Read the model definition and answer for the solid it produces. Units are mm, in the model's axes. A direction names the side the tool comes from. Round coordinates to 2 decimals unless told otherwise and drop trailing zeros. Order: outer loops, then holes, each group sorted by start corner. A loop starts at its lowest first (then second) coordinate and runs counter-clockwise, first axis right, second up. Notation, with made-up numbers: (-18.75, 35.25) -> (36.25, 35.25) arc R12 ccw to (36.25, 58.25) -> close; hole circle Ø8 at (53.5, -26.75). An arc over 180 degrees is marked (long way). Answer as a JSON object with one key per item and string values. Group by question number.
Item 1: Section D-D, the plane x = 59 is taken. Write down the section's boundary in (y, z).
Item 2: Section A-A, the plane z = 55 is taken. Write down the section's boundary in (x, y).
Item 3: Given P1, Ø2.5, axis at y = -5.1, z = 46.17, coming from the -X side; P2, Ø3, axis at x = -16.5, y = 42.5, coming from the -Z side; P3, Ø3, axis at x = -42.5, y = -17.6, coming from the +Z side, each flat-ended and moving along its own axis, determine where each tip first touches the part or whether it passes through.
Item 4: For faces 1 (the flat face through (16, 43, 2)), 2 (the cylindrical face through (-49, -48, 3)), 3 (the flat face through (85, -1, 76)), determine the directions among +Z, -Z, +X, -X, +Y, -Y from which every point of the face is accessible in a straight line to the end or side of a thin tool.
Item 5: Section C-C, the plane x = -25.5 is taken. Write down the section's boundary in (y, z).
Item 6: Section B-B, the plane x = 0 is taken. Write down the section's boundary in (y, z), plus the area to 3 significant figures.
Item 7: The mould has two halves that part along Z. Classify faces 4 (the flat face through (87, 1, 105)), 5 (the flat face through (-42, 16, 2)), 6 (the cylindrical face through (18.25, 39.57, 0.99)), 7 (the cylindrical face through (87.5, -4.3, 62)): pulls with the +Z half, pulls with the -Z half, needs draft (parallel to the pull), parting line crosses it, or undercut.
Item 8: Consider probe 1 along Y at (x, z) = (87, 55); probe 2 along Z at (x, y) = (47, -35); probe 3 along X at (y, z) = (-45.5, 28.5). Determine where each line is inside the solid, lowest interval first. Write a range as from..to.
Autodesk Inventor part; units mm, degrees
ref_plane "YZ Plane" through (0, 0, 0) normal (1, 0, 0) x (0, 1, 0)
ref_plane "XZ Plane" through (0, 0, 0) normal (0, 1, 0) x (-1, 0, 0)
ref_plane "XY Plane" through (0, 0, 0) normal (0, 0, 1) x (1, 0, 0)
sketch "スケッチ1" plane through (0, 0, 0) normal (0, 0, 1) x (1, 0, 0)
  circle A0 centre (0, 0) radius 48.5
  circle A1 centre (0, 0) radius 46.0893
  line L0 (-50, 50) -> (50, 50)
  line L1 (50, 50) -> (50, -50)
  line L2 (50, -50) -> (-50, -50)
  line L3 (-50, -50) -> (-50, 50)
  dimension "d0" = 97
  dimension "d3" = 50
  dimension "d4" = 50
  dimension "d5" = 50
  dimension "d6" = 50
extrude "押し出し1" add sketch "スケッチ1" along normal blind 5 contours A0 | A1 | L0 L1 L2 L3
sketch "スケッチ2" plane through (0, 0, 5) normal (0, 0, 1) x (1, 0, 0)
  circle A0 centre (0, 0) radius 46
  line L0 (0, 0) -> (0, 64.6511)
  line L1 (0, 0) -> (-25.9524, 62.6547)
  line L2 (-50, 50) -> (-50, -50)
  point P0 (-17.6034, 42.4985)
  point P1 (-42.4985, 17.6034)
  point P2 (-42.4985, -17.6034)
  point P3 (-17.6034, -42.4985)
  point P4 (17.6034, -42.4985)
  point P5 (42.4985, -17.6034)
  point P6 (42.4985, 17.6034)
  point P7 (17.6034, 42.4985)
  dimension "d7" = 92
  dimension "d8" = 22.5
  dimension "d11" = 360
  dimension "d76" = 50
hole "穴1" at (-17.6034, 42.4985, 5) at (-42.4985, 17.6034, 5) at (-42.4985, -17.6034, 5) at (-17.6034, -42.4985, 5) at (17.6034, -42.4985, 5) at (42.4985, -17.6034, 5) at (42.4985, 17.6034, 5) at (17.6034, 42.4985, 5) direction (0, 0, -1) diameter 2.459 end through all
sketch "スケッチ3" plane through (0, 0, 5) normal (0, 0, 1) x (1, 0, 0)
  circle A0 centre (0, 0) radius 30
  dimension "d20" = 60
extrude "押し出し2" cut sketch "スケッチ3" against normal blind 5
sketch "スケッチ4" plane through (50, -50, 0) normal (1, 0, 0) x (0, 0, -1)
  line L0 (-5, 100) -> (-5, 0)
  line L1 (-5, 100) -> (0, 100)
  line L2 (0, 100) -> (0, 0)
  line L3 (0, 0) -> (-5, 0)
  line L4 (-5, 0) -> (-5, 100)
  point P0 (0, 50)
extrude "押し出し3" add sketch "スケッチ4" along normal blind 40
sketch "スケッチ5" plane through (0, 0, 5) normal (0, 0, 1) x (1, 0, 0)
  line L0 (-50, 50) -> (90, 50)
  line L1 (85, 50) -> (90, 50)
  line L2 (90, 50) -> (90, -50)
  line L3 (90, -50) -> (85, -50)
  line L4 (85, -50) -> (85, 50)
  line L5 (-50, -50) -> (90, -50)
  line L6 (90, 50) -> (90, -50)
  point P0 (0, 0)
  point P1 (90, 50)
  point P2 (90, 0)
  dimension "d25" = 0
  dimension "d26" = 5
  dimension "d27" = 100
  dimension "d70" = 0
extrude "押し出し4" add sketch "スケッチ5" along normal blind 100
sketch "スケッチ6" plane through (90, -50, 0) normal (1, 0, 0) x (0, 0, -1)
  circle A0 centre (-55, 50) radius 46
  line L0 (0, 0) -> (-105, 0)
  line L1 (0, 0) -> (0, 100)
  line L2 (-55, 50) -> (41.9537, 50)
  line L3 (-55, 50) -> (-55, 131.7305)
  line L4 (-55, 50) -> (-80.0101, 110.3797)
  circle A1 centre (-55, 50) radius 12.5
  line L5 (-55, 50) -> (-63.1841, 64.1753)
  point P0 (0, 50)
  point P1 (-72.6034, 92.4985)
  point P2 (-97.4985, 67.6034)
  point P3 (-97.4985, 32.3966)
  point P4 (-72.6034, 7.5015)
  point P5 (-37.3966, 7.5015)
  point P6 (-12.5015, 32.3966)
  point P7 (-12.5015, 67.6034)
  point P8 (-37.3966, 92.4985)
  point P9 (-61.25, 60.8253)
  point P10 (-67.5, 50)
  point P11 (-61.25, 39.1747)
  point P12 (-48.75, 39.1747)
  point P13 (-42.5, 50)
  point P14 (-48.75, 60.8253)
  dimension "d32" = 92
  dimension "d34" = 25
  dimension "d30" = 50
  dimension "d31" = 55
  dimension "d33" = 22.5
  dimension "d35" = 30
  dimension "d38" = 360
  dimension "d42" = 360
hole "穴2" at (90, 10.8253, 48.75) at (90, 10.8253, 61.25) at (90, 0, 67.5) at (90, 0, 42.5) at (90, -10.8253, 48.75) at (90, -10.8253, 61.25) direction (-1, 0, 0) diameter 2.459 end through all
sketch "スケッチ7" plane through (90, -50, 0) normal (1, 0, 0) x (0, 0, -1)
  line L0 (-55, 50) -> (26.223, 50)
  circle A0 centre (-55, 50) radius 10.2
  line L1 (0, 0) -> (0, 100)
  line L2 (0, 0) -> (-105, 0)
  line L3 (-55, 50) -> (-55, 82.0983)
  point P0 (0, 50)
  point P1 (-55, 60.2)
  point P2 (-63.8335, 44.9)
  point P3 (-46.1665, 44.9)
  dimension "d53" = 20.4
  dimension "d51" = 55
  dimension "d52" = 50
  dimension "d56" = 360
hole "穴3" at (90, 10.2, 55) at (90, -5.1, 63.8335) at (90, -5.1, 46.1665) direction (-1, 0, 0) diameter 4 end through all
sketch "スケッチ8" plane through (90, -50, 0) normal (1, 0, 0) x (0, 0, -1)
  circle A0 centre (-55, 50) radius 6.5
  line L0 (0, 0) -> (0, 100)
  line L1 (0, 0) -> (-105, 0)
  point P0 (0, 50)
  dimension "d65" = 13
  dimension "d66" = 55
  dimension "d67" = 50
extrude "押し出し5" cut sketch "スケッチ8" against normal through all
sketch "スケッチ13" plane through (0, 0, 0) normal (0, 1, 0) x (-1, 0, 0)
  line L0 (-90, 0) -> (-50, 0)
  line L1 (-50, 0) -> (-50, 30)
  line L2 (-50, 30) -> (-90, 30)
  line L3 (-90, 30) -> (-90, 0)
  line L4 (-90, 0) -> (-90, 105)
  line L5 (50, 0) -> (-90, 0)
  arc A0 (-85, 10) -> (-80, 5) centre (-80, 10) ccw
  line L6 (-80, 5) -> (-46.2653, 5)
  line L7 (-50, 5) -> (-85, 30)
  point P0 (0, 0)
  point P1 (-90, 5)
  point P2 (-90, 100)
  point P3 (45, 0)
  point P4 (-85, 0)
  dimension "d92" = 40
  dimension "d93" = 0
  dimension "d94" = 30
  dimension "d95" = 0
extrude "押し出し9" add sketch "スケッチ13" along normal mid plane 100 contours L3 L2 L7 L1 L0
fillet "フィレット2" radius 5 7 edges at (-50, -50, 2.5) (-50, 50, 2.5) (85, 0, 30) (90, 0, 0) (50, 0, 5) (87.5, -50, 105) (87.5, 50, 105)
sketch "スケッチ16" plane through (0, 0, 0) normal (0, 0, -1) x (-1, 0, 0)
  circle A0 centre (17.6034, 42.4985) radius 1.2295
  circle A1 centre (0, 0) radius 46
  circle A2 centre (17.6034, 42.4985) radius 3
  circle A3 centre (-17.6034, 42.4985) radius 3
  circle A4 centre (-42.4985, 17.6034) radius 3
  circle A5 centre (-42.4985, -17.6034) radius 3
  circle A6 centre (-17.6034, -42.4985) radius 3
  circle A7 centre (17.6034, -42.4985) radius 3
  circle A8 centre (42.4985, -17.6034) radius 3
  circle A9 centre (42.4985, 17.6034) radius 3
  dimension "d113" = 6
  dimension "d116" = 360
extrude "押し出し12" cut sketch "スケッチ16" against normal blind 2 contours A0 A1 | A0 A1 A2 | A1 A0 | A0 A1 A2 | A3 A1 | A1 A3 | A9 A1 | A1 A9 | A4 A1 | A1 A4 | A8 A1 | A1 A8 | A5 A1 | A1 A5 | A7 A1 | A1 A7 | A6 A1 | A1 A6
properties part number "legparts_07(four)"
Values found:
{
 "1": {"outline": "(-50, 0) -> (50, 0) -> (50, 11.43) -> (-50, 11.43) -> close"},
 "2": {"outline": "(85, -50) -> (90, -50) -> (90, -6.5) -> (85, -6.5) -> close; (85, 6.5) -> (90, 6.5) -> (90, 8.2) -> (85, 8.2) -> close; (85, 12.2) -> (90, 12.2) -> (90, 50) -> (85, 50) -> close"},
 "3": {"P1": "through", "P2": "z = 2", "P3": "z = 5"},
 "4": {"face 1": "-Z", "face 2": "+Z, -Z, -X, -Y", "face 3": "+Z, -X, +Y, -Y"},
 "5": {"outline": "(-50, 0) -> (-15.8, 0) -> (-15.8, 5) -> (-50, 5) -> close; (15.8, 0) -> (50, 0) -> (50, 5) -> (15.8, 5) -> close"},
 "6": {"outline": "(-50, 0) -> (-30, 0) -> (-30, 5) -> (-50, 5) -> close; (30, 0) -> (50, 0) -> (50, 5) -> (30, 5) -> close", "area": "200 mm2"},
 "7": {"face 4": "pulls with the +Z half", "face 5": "pulls with the -Z half", "face 6": "needs draft", "face 7": "undercut"},
 "8": {"probe 1": "-50..-6.5, 6.5..8.2, 12.2..50", "probe 2": "0..5", "probe 3": "82.9..90"}
}
